Design review of the part built by this model. Coordinates are the model's own, in mm. Face numbers are marked on the shaded views. A direction names the side the tool comes from. Give positions to 0.01 mm unless a question says otherwise; leave off trailing zeros. Loops run counter-clockwise (first coordinate to the right, second up) from the corner with the lowest first, then second, coordinate; pieces in that order, holes last. Notation, with made-up numbers: (83.25, 47.25) -> (132.25, 47.25) arc R27 ccw to (132.25, 69.25) -> close; hole circle Ø11 at (48, 28). An arc over 180 degrees is marked (long way). Answer in a Markdown table with one row per item. Add a question column.
(1) For the marked faces 4 and 5, list the 3-axis set-ups (+Z, -Z, +X, -X, +Y, -Y) from which the entire face can be reached by the end or side of a thin tool; tool diameter is ignored.
(2) Consider section D-D on x = 113.5. Write out the cut boundary in (y, z).
(3) Consider section A-A on x = -574. Write out the cut boundary in (y, z), then the cut area to 3 significant figures.
(4) For line 1 (X direction, y = 75.5, z = -654); line 2 (Y direction, x = 104, z = -506.5), list the stretches that pass through material, from the lowest coordinate up.
(5) For pin 1 (1 mm diameter, centred on x = -153, y = 76.5, fed in from -Z), flat-tipped, find the tip position at first contact; note if it passes through.
(6) Consider section B-B on y = 196. Write out the cut boundary in (x, z), then the cut area to 3 significant figures.
(7) Consider section C-C on z = -365. Write out the cut boundary in (x, y).
(8) Draft analysis for pull direction Y (two halves, no side actions). For the marked faces 1, 2 and 3, state which applies: +Y half, -Y half, draft (parallel to the pull), parting line (faces both ways), or undercut.
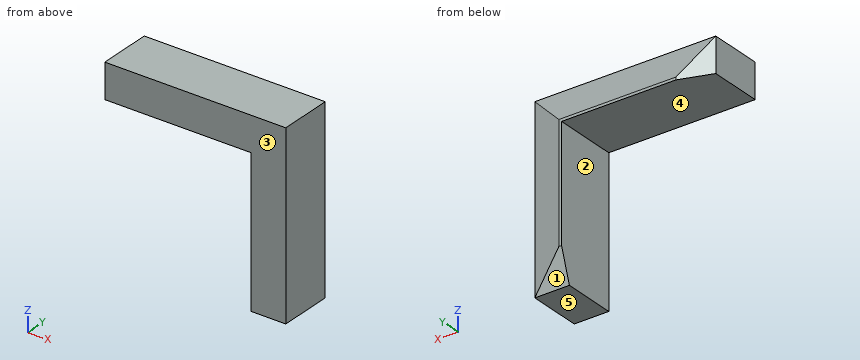
Autodesk Inventor part; units mm, degrees
ref_plane "YZ Plane" through (0, 0, 0) normal (1, 0, 0) x (0, 1, 0)
ref_plane "XZ Plane" through (0, 0, 0) normal (0, 1, 0) x (-1, 0, 0)
ref_plane "XY Plane" through (0, 0, 0) normal (0, 0, 1) x (1, 0, 0)
sketch "Sketch1" plane through (0, 0, 0) normal (0, 1, 0) x (-1, 0, 0)
  line L0 (0, 0) -> (698.5, 0)
  line L1 (0, 0) -> (0, -698.5)
  line L2 (0, -698.5) -> (-165.1, -698.5)
  line L3 (698.5, 0) -> (698.5, 165.1)
  line L4 (-165.1, -698.5) -> (-165.1, 165.1)
  line L5 (-165.1, 165.1) -> (698.5, 165.1)
  dimension "d1" = 698.5
  dimension "d2" = 698.5
  dimension "d3" = 165.1
  dimension "d4" = 165.1
  dimension "d5" = 863.6
  dimension "d6" = 863.6
extrude "Extrusion1" add sketch "Sketch1" along normal blind 304.8
sketch "Sketch2" plane through (-698.5, 0, 0) normal (-1, 0, 0) x (0, 0, 1)
  line L0 (0, 304.8) -> (165.1, 304.8)
  line L1 (165.1, 0) -> (165.1, 304.8)
  line L2 (12.7, 304.8) -> (165.1, 254)
  line L3 (165.1, 254) -> (165.1, 304.8)
  line L4 (165.1, 304.8) -> (12.7, 304.8)
  point P0 (0, 0)
  dimension "d9" = 12.7
  dimension "d10" = 50.8
sketch3d "3D Sketch1"
  line L0 (-698.5, 304.8, 0) -> (0, 304.8, 0)
  line L1 (0, 304.8, 0) -> (0, 304.8, -698.5)
sweep "Sweep1" cut profiles "Sketch2" path "3D Sketch1"
sketch "Sketch3" plane through (0, 0, 0) normal (0, 0, -1) x (-1, 0, 0)
  line L0 (698.5, 304.8) -> (-12.7, 304.8)
  line L1 (698.5, 254) -> (698.5, 304.8)
  line L2 (698.5, 0) -> (698.5, 254)
  line L3 (546.1, 304.8) -> (698.5, 254)
  line L4 (698.5, 254) -> (698.5, 304.8)
  line L5 (698.5, 304.8) -> (546.1, 304.8)
  point P0 (0, 0)
  dimension "d13" = 152.4
  dimension "d14" = 50.8
extrude "Extrusion2" cut sketch "Sketch3" against normal through all
sketch "Sketch4" plane through (0, 0, -698.5) normal (-1, 0, 0) x (0, 0, 1)
  line L0 (0, 304.8) -> (698.5, 304.8)
  line L1 (0, 304.8) -> (0, 254)
  line L2 (0, 254) -> (152.4, 304.8)
  line L3 (152.4, 304.8) -> (0, 304.8)
  line L4 (0, 304.8) -> (0, 254)
  point P0 (698.5, 0)
  point P1 (0, 254)
  dimension "d17" = 152.4
  dimension "d18" = 50.8
extrude "Extrusion3" cut sketch "Sketch4" against normal through all
equation "\"d2\" = d1"
equation "\"d4\" = d3"
properties part number "Corner_cap_5" material "Limestone"
Values follow:
| question | item | result |
|---|---|---|
| 1 | face 4 | -Z, -X, +Y, -Y |
| 1 | face 5 | -Z, +X, -X, +Y, -Y |
| 2 | outline | (0, -698.5) -> (254, -698.5) -> (271.2, -646.9) -> (271.2, 113.5) -> (254, 165.1) -> (0, 165.1) -> close |
| 3 | outline | (0, 0) -> (295.5, 0) -> (295.5, 40.6) -> (254, 165.1) -> (0, 165.1) -> close |
| 3 | area | 46,200 mm2 |
| 4 | line 1 | 0 to 165.1 |
| 4 | line 2 | 0 to 274.37 |
| 5 | pin 1 | z = 0 |
| 6 | outline | (-698.5, 0) -> (0, 0) -> (0, -698.5) -> (165.1, -698.5) -> (165.1, 165.1) -> (-698.5, 165.1) -> close |
| 6 | area | 258,000 mm2 |
| 7 | outline | (0, 0) -> (165.1, 0) -> (165.1, 254) -> (12.7, 304.8) -> (0, 304.8) -> close |
| 8 | face 1 | +Y half |
| 8 | face 2 | draft |
| 8 | face 3 | -Y half |
